from build123d import *

# Parameters (mm, degrees)
F0_R     = 27
F0_R_2   = 3
F1_DEPTH = 3
F3_DEPTH = 3
F4_R     = 3


# Not quite as in the source:
# - a feature names something its author has since deleted; it is built from what else it names


with BuildPart() as f1:
    # F0 (on Front) → F1 (new body)
    with BuildSketch(Plane.XZ):
        Circle(F0_R)
        Circle(F0_R_2, mode=Mode.SUBTRACT)
    extrude(amount=F1_DEPTH)

    # F2 (on face) → F3 (cut)
    with BuildSketch(Plane.XZ.offset(3)):
        with BuildLine():
            Line((-9.2, 30.5910954097), (-9.2, 18))
            ThreePointArc((-9.2, 18), (0, 8.8), (9.2, 18))
            Line((9.2, 18), (9.2, 30.5910954097))
            Line((9.2, 30.5910954097), (-9.2, 30.5910954097))
        make_face()
    extrude(amount=-F3_DEPTH, mode=Mode.SUBTRACT)

    # F4
    f4_edges = [f1.edges().sort_by_distance(p)[0] for p in [
        (-9.2, -1.5, 25.384247),
        (9.2, -1.5, 25.384247),
    ]]
    fillet(f4_edges, radius=F4_R)


solid = f1.part
Verification items for the finished model (mm, model axes). A direction names the side the tool comes from. Coordinates: 2 decimals unless noted, no trailing zeros. Order: outer loops, then holes, each group sorted by start corner. A loop starts at its lowest first (then second) coordinate and runs counter-clockwise, first axis right, second up. Notation, with made-up numbers: M -39,-35.75 L -10,-35.75 A24 cw -10,-8.75 Z; hole C 23,-14 d11. An arc over 180 degrees is marked long. One line per item, written item: value. Start each with the question number.
Item 1: Sectioned sample at C-C (y = -2). Enter the section's corners in (x, z) (3 decimals).
Item 2: Access from +Z, -Z, +X, -X, +Y, -Y to the whole of each face (thin tool, end or side, straight path). Record for faces 1 (the cylindrical face through (-0.99, -1.48, -26.98)), 2 (the flat face through (9.2, -2, 19)).
Item 3: Sectioned sample at B-B (z = 0). Enter the section's corners in (x, y).
Item 4: Gauge pin test, flat ends, axial feed: pin 1 (0.8 mm diameter, centred on y = -2, z = 19.5, fed in from +X); pin 2 (1 mm diameter, centred on x = 18, y = -2, fed in from +Z); pin 3 (0.8 mm diameter, centred on y = -2, z = 19, fed in from -X). Record the tip position at first contact, or that the pin passes through.
Item 5: Sectioned sample at D-D (z = -7). Enter the section's corners in (x, y).
Item 6: Scan lines: probe 1 along Z at (x, y) = (0, -1.9); probe 2 along X at (y, z) = (-0.2, 9.5); probe 3 along X at (y, z) = (-2.6, 16.5). Record each from-to range of solid material in increasing order.
Item 7: Mould release check, pull along Z, two halves, no side actions. Record for faces 3 (the cylindrical face through (-3, -1, 0)), 4 (the cylindrical face through (-10.751, -1.479, 23.295)), 5 (the flat face through (0, 0, -7)): released by +Z, released by -Z, zero draft, split by the parting line, or undercut.
Item 8: Sectioned sample at A-A (x = 0). Enter the section's corners in (y, z).
Conclusion:
1. outline: M -13.725,23.251 A27 ccw long 13.725,23.251 A3 ccw 9.2,20.668 L 9.2,18 A9.2 cw -9.2,18 L -9.2,20.668 A3 ccw Z; hole C 0,0 d6
2. face 1: +Y, -Y
2. face 2: +Z, +Y, -Y
3. outline: M -27,-3 L -3,-3 L -3,0 L -27,0 Z; M 3,-3 L 27,-3 L 27,0 L 3,0 Z
4. pin 1: stops at x = 19.08
4. pin 2: stops at z = 20.56
4. pin 3: stops at x = -19.57
5. outline: M -26.08,-3 L 26.08,-3 L 26.08,0 L -26.08,0 Z
6. probe 1: z = -27 to -3, 3 to 8.8
6. probe 2: x = -25.27 to -3.52, 3.52 to 25.27
6. probe 3: x = -21.37 to -9.08, 9.08 to 21.37
7. face 3: undercut
7. face 4: released by +Z
7. face 5: zero draft
8. outline: M -3,-27 L 0,-27 L 0,-3 L -3,-3 Z; M -3,3 L 0,3 L 0,8.8 L -3,8.8 Z
